```python
from build123d import *

# Parameters (mm, degrees)
SKETCH_1_W          = 68
SKETCH_1_H          = 27
EXTRUDE_1_DEPTH     = 11
SKETCH_2_W          = 63.5
SKETCH_2_H          = 22.5
CUT_EXTRUDE_1_DEPTH = 9.5
CUT_EXTRUDE_2_DEPTH = 2.25
SKETCH_4_W          = 21.5
SKETCH_4_H          = 9.5
CUT_EXTRUDE_3_DEPTH = 2.25
EXTRUDE_2_DEPTH     = 9.5
EXTRUDE_3_DEPTH     = 9.5
SKETCH_7_R          = 1
CUT_EXTRUDE_4_DEPTH = 9.5
FILLET_1_R          = 2


with BuildPart() as part:
    # Эскиз1 → Бобышка-Вытянуть1 (new body)
    with BuildSketch(Plane(origin=(0, 0, 0), x_dir=(1, 0, 0), z_dir=(0, 1, 0))):
        Rectangle(SKETCH_1_W, SKETCH_1_H)
    extrude(amount=EXTRUDE_1_DEPTH)

    # Эскиз2 → Вырез-Вытянуть1 (cut)
    with BuildSketch(Plane.XZ):
        Rectangle(SKETCH_2_W, SKETCH_2_H)
    extrude(amount=-CUT_EXTRUDE_1_DEPTH, mode=Mode.SUBTRACT)

    # Эскиз3 → Вырез-Вытянуть2 (cut)
    with BuildSketch(Plane.ZY.offset(34)):
        with BuildLine():
            Line((-4.6, 2.1), (-4.6, 0))
            Line((-4.6, 0), (4.6, 0))
            Line((4.6, 0), (4.6, 2.1))
            ThreePointArc((4.6, 2.1), (4.219238816, 3.019238816), (3.3, 3.4))
            Line((3.3, 3.4), (-3.3, 3.4))
            ThreePointArc((-3.3, 3.4), (-4.219238816, 3.019238816), (-4.6, 2.1))
        make_face()
    extrude(amount=-CUT_EXTRUDE_2_DEPTH, mode=Mode.SUBTRACT)

    # Эскиз4 → Вырез-Вытянуть3 (cut)
    with BuildSketch(Plane(origin=(34, 0, 0), x_dir=(0, 0, -1), z_dir=(1, 0, 0))):
        with Locations((0, 4.75)):
            Rectangle(SKETCH_4_W, SKETCH_4_H)
    extrude(amount=-CUT_EXTRUDE_3_DEPTH, mode=Mode.SUBTRACT)

    # Эскиз5 → Бобышка-Вытянуть2 (add)
    with BuildSketch(Plane.XZ.offset(-9.5)):
        with BuildLine():
            Line((-19.5, -9), (-19.5, -11.25))
            Line((-19.5, -11.25), (-23.5, -11.25))
            Line((-23.5, -11.25), (-23.5, -9))
            ThreePointArc((-23.5, -9), (-21.5, -7), (-19.5, -9))
        make_face()
        with BuildLine():
            Line((-23.5, 11.25), (-23.5, 9))
            ThreePointArc((-23.5, 9), (-21.5, 7), (-19.5, 9))
            Line((-19.5, 9), (-19.5, 11.25))
            Line((-19.5, 11.25), (-23.5, 11.25))
        make_face()
    extrude(amount=EXTRUDE_2_DEPTH)

    # Эскиз6 → Бобышка-Вытянуть3 (add)
    with BuildSketch(Plane.XZ.offset(-9.5)):
        with BuildLine():
            Line((23.7, -11), (23.7, -11.25))
            Line((23.7, -11.25), (22.3, -11.25))
            Line((22.3, -11.25), (22.3, -11))
            ThreePointArc((22.3, -11), (23, -10.3), (23.7, -11))
        make_face()
        with BuildLine():
            Line((22.3, 11.25), (22.3, 11))
            ThreePointArc((22.3, 11), (23, 10.3), (23.7, 11))
            Line((23.7, 11), (23.7, 11.25))
            Line((23.7, 11.25), (22.3, 11.25))
        make_face()
    extrude(amount=EXTRUDE_3_DEPTH)

    # Эскиз7 → Вырез-Вытянуть4 (cut)
    with BuildSketch(Plane.XZ):
        with Locations(Location((-21.5, -9, 0), (0, 0, 270))):
            Circle(SKETCH_7_R)
        with Locations(Location((-21.5, 9, 0), (0, 0, 270))):
            Circle(SKETCH_7_R)
    extrude(amount=-CUT_EXTRUDE_4_DEPTH, mode=Mode.SUBTRACT)

    # Скругление1
    # the kernel refuses this fillet: 2 mm, written as the material it takes off along each edge
    with BuildSketch(Plane(origin=(32, 9, -11.5), x_dir=(1, 0, 0), z_dir=(0, 0, -1))) as fillet_1_piece_1_section:
        Polygon((0, 0), (FILLET_1_R, 0), (FILLET_1_R, -FILLET_1_R), (0, -FILLET_1_R), align=None)
    fillet_1_piece_1 = extrude(amount=FILLET_1_R, mode=Mode.PRIVATE)
    fillet_1_piece_1 = fillet_1_piece_1 - Plane(origin=(32, 9, -11.5), x_dir=(-0.7071067811865475, -0.7071067811865475, 0), z_dir=(0, 0, -1)) * Sphere(FILLET_1_R, mode=Mode.PRIVATE)
    add(fillet_1_piece_1, mode=Mode.SUBTRACT)
    with BuildSketch(Plane(origin=(32, 9, 11.5), x_dir=(0, 0, 1), z_dir=(1, 0, 0))) as fillet_1_piece_2_section:
        Polygon((0, 0), (FILLET_1_R, 0), (FILLET_1_R, -FILLET_1_R), (0, -FILLET_1_R), align=None)
    fillet_1_piece_2 = extrude(amount=FILLET_1_R, mode=Mode.PRIVATE)
    fillet_1_piece_2 = fillet_1_piece_2 - Plane(origin=(32, 9, 11.5), x_dir=(0, -0.7071067811865475, -0.7071067811865475), z_dir=(1, 0, 0)) * Sphere(FILLET_1_R, mode=Mode.PRIVATE)
    add(fillet_1_piece_2, mode=Mode.SUBTRACT)
    with BuildSketch(Plane(origin=(-32, 9, 11.5), x_dir=(0, 0, 1), z_dir=(-1, 0, 0))) as fillet_1_piece_3_section:
        Polygon((0, 0), (FILLET_1_R, 0), (FILLET_1_R, FILLET_1_R), (0, FILLET_1_R), align=None)
    fillet_1_piece_3 = extrude(amount=FILLET_1_R, mode=Mode.PRIVATE)
    fillet_1_piece_3 = fillet_1_piece_3 - Plane(origin=(-32, 9, 11.5), x_dir=(0, -0.7071067811865475, -0.7071067811865475), z_dir=(-1, 0, 0)) * Sphere(FILLET_1_R, mode=Mode.PRIVATE)
    add(fillet_1_piece_3, mode=Mode.SUBTRACT)
    with BuildSketch(Plane(origin=(-32, 9, -11.5), x_dir=(-1, 0, 0), z_dir=(0, 0, -1))) as fillet_1_piece_4_section:
        Polygon((0, 0), (FILLET_1_R, 0), (FILLET_1_R, FILLET_1_R), (0, FILLET_1_R), align=None)
    fillet_1_piece_4 = extrude(amount=FILLET_1_R, mode=Mode.PRIVATE)
    fillet_1_piece_4 = fillet_1_piece_4 - Plane(origin=(-32, 9, -11.5), x_dir=(0.7071067811865475, -0.7071067811865475, 0), z_dir=(0, 0, -1)) * Sphere(FILLET_1_R, mode=Mode.PRIVATE)
    add(fillet_1_piece_4, mode=Mode.SUBTRACT)
    with BuildSketch(Plane(origin=(34, 11, -11.5), x_dir=(0, -1, 0), z_dir=(0, 0, 1)), Plane(origin=(-34, 11, 11.5), x_dir=(0, -1, 0), z_dir=(0, 0, -1))) as fillet_1_piece_5:
        with BuildLine():
            CenterArc((FILLET_1_R, -FILLET_1_R), FILLET_1_R, 90, 90)
            Line((0, -FILLET_1_R), (0, 0))
            Line((0, 0), (FILLET_1_R, 0))
        make_face()
    extrude(amount=23, mode=Mode.SUBTRACT)
    with BuildSketch(Plane(origin=(34, -5, 13.5), x_dir=(0, 0, -1), z_dir=(0, 1, 0)), Plane(origin=(34, -5, -13.5), x_dir=(-1, 0, 0), z_dir=(0, 1, 0))) as fillet_1_piece_6:
        with BuildLine():
            CenterArc((FILLET_1_R, FILLET_1_R), FILLET_1_R, 180, 90)
            Line((0, FILLET_1_R), (0, 0))
            Line((0, 0), (FILLET_1_R, 0))
        make_face()
    extrude(amount=14, mode=Mode.SUBTRACT)
    with BuildSketch(Plane(origin=(32, 11, 13.5), x_dir=(0, 0, -1), z_dir=(-1, 0, 0))) as fillet_1_piece_7:
        with BuildLine():
            CenterArc((FILLET_1_R, FILLET_1_R), FILLET_1_R, 180, 90)
            Line((0, FILLET_1_R), (0, 0))
            Line((0, 0), (FILLET_1_R, 0))
        make_face()
    extrude(amount=64, mode=Mode.SUBTRACT)
    with BuildSketch(Plane(origin=(-34, -5, 13.5), x_dir=(0, 0, -1), z_dir=(0, 1, 0)), Plane(origin=(-34, -5, -13.5), x_dir=(1, 0, 0), z_dir=(0, 1, 0))) as fillet_1_piece_8:
        with BuildLine():
            CenterArc((FILLET_1_R, -FILLET_1_R), FILLET_1_R, 90, 90)
            Line((0, -FILLET_1_R), (0, 0))
            Line((0, 0), (FILLET_1_R, 0))
        make_face()
    extrude(amount=14, mode=Mode.SUBTRACT)
    with BuildSketch(Plane(origin=(-32, 11, -13.5), x_dir=(0, -1, 0), z_dir=(1, 0, 0))) as fillet_1_piece_9:
        with BuildLine():
            CenterArc((FILLET_1_R, -FILLET_1_R), FILLET_1_R, 90, 90)
            Line((0, -FILLET_1_R), (0, 0))
            Line((0, 0), (FILLET_1_R, 0))
        make_face()
    extrude(amount=64, mode=Mode.SUBTRACT)


solid = part.part
```
Work out the finished part from the listing and answer in its coordinate system (mm). A direction names the side the tool comes from. Coordinates: 2 decimals unless noted, no trailing zeros. Loops run counter-clockwise (first coordinate to the right, second up) from the corner with the lowest first, then second, coordinate; pieces in that order, holes last.
1) Flat-ended cylindrical pins translate along their axes: pin 1 (1 mm diameter, centred on x = -17.5, z = 5.5, fed in from -Y); pin 2 (1.1 mm diameter, centred on x = -33, z = -1.5, fed in from -Y). Find the tip coordinate at first contact, or state that the pin passes through.
Results:
pin 1: stops at y = 9.5
pin 2: stops at y = 3.4
2) Section B-B (x = -21.5) is taken. Give the vertices of the cut face in (y, z), plus the area to 3 significant figures.
Results:
outline: (0, -13.5) - (9, -13.5) arc R2 ccw to (11, -11.5) - (11, 11.5) arc R2 ccw to (9, 13.5) - (0, 13.5) - (0, 10) - (9.5, 10) - (9.5, 8) - (0, 8) - (0, 7) - (9.5, 7) - (9.5, -7) - (0, -7) - (0, -8) - (9.5, -8) - (9.5, -10) - (0, -10) - close
area: 124 mm2
3) For a pull along X with two mould halves and no side action, classify faces 6 (the cylindrical face through (-33.43, 4.44, 12.9)), 7 (the flat face through (-28, 5, 11.25)), 8 (the cylindrical face through (-0.45, 10.4, -12.93)) as +X half, -X half, draft (parallel to the pull), parting line (faces both ways), or undercut.
Results:
face 6: -X half
face 7: undercut
face 8: draft
4) Section A-A (z = -5.5) is taken. Give the vertices of the cut face in (x, y), plus the area to 3 significant figures.
Results:
outline: (-34, 0) - (-31.75, 0) - (-31.75, 9.5) - (33.94, 9.5) arc R2 ccw to (32, 11) - (-32, 11) arc R2 ccw to (-34, 9) - close
area: 122 mm2
5) Section C-C (y = 6.75) is taken. Give the number of separate pieces and of enclosed holes in the cut face, plus the area to 3 significant figures.
Results:
separate pieces: 1
enclosed holes: 2
area: 382 mm2
6) Consider probe 1 along X at (y, z) = (3.5, 9); probe 2 along X at (y, z) = (3.25, -9.5); probe 3 along X at (y, z) = (4.75, 4.75). Determine where each line is inside the solid, lowest interval first.
Results:
probe 1: x = -34 to -31.75, -23.5 to -22.5, -20.5 to -19.5
probe 2: x = -34 to -31.75, -23.5 to -22.37, -20.63 to -19.5
probe 3: x = -34 to -31.75
7) For faces 1 (the flat face through (1, 5, -11.25)), 2 (the cylindrical face through (-33.43, 10.4, 0.16)), 3 (the flat face through (-33, 1, -4.6)), 4 (the flat face through (33, 5, -10.75)), 5 (the flat face through (0, 11, 0)), determine the directions among +Z, -Z, +X, -X, +Y, -Y from which every point of the face is accessible in a straight line to the end or side of a thin tool.
Results:
face 1: -Y
face 2: +Z, -Z, -X, +Y
face 3: +X, -X, -Y
face 4: +X, -Y
face 5: +Z, -Z, +X, -X, +Y
